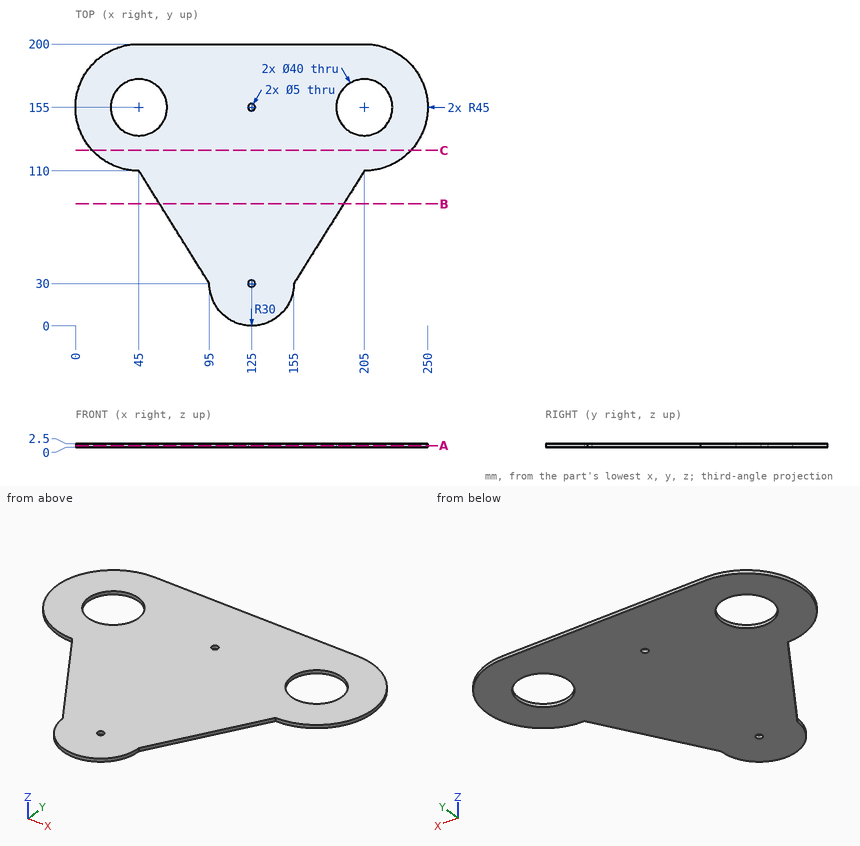
Source: three-view drawing plus pictorial views. Frame: mm from the lowest corner of the part. Round coordinates to 2 decimals unless told otherwise and drop trailing zeros. Write each loop counter-clockwise with the first axis right and the second up, starting at its lowest first coordinate (ties: lowest second). Pieces come first, ordered by that corner, then holes. Notation, with made-up numbers: M 63.5,27 L 72.5,27 A10 ccw 72.5,42 Z; hole C -22,-23 d3. An arc over 180 degrees is marked long. Use CSV: the item, a comma, the result in double quotes. Start each with the question number.
Q1. Cut plane C-C on y = 124.5. Output: boundary loops of the cut face in (x, z).
Q2. Line query: line 1 (Y direction, x = 125, z = 0.8); line 2 (Y direction, x = 206.5, z = 1.7) (3 decimals); line 3 (X direction, y = 169.5, z = 2.25). Output: solid intervals per line, ascending. Write a range as from..to.
Q3. Cut plane A-A on z = 1.25. Output: boundary loops of the cut face in (x, y), plus the area to 3 significant figures.
Q4. First-contact query: P1, Ø1.5, axis at x = 224.5, z = 0.5, coming from the -Y side; P2, Ø1.5, axis at x = 221, z = 2, coming from the +Y side. Flat tips, straight axial feed; report the tip coordinate or a pass-through.
Q5. Cut plane B-B on y = 86.5. Output: boundary loops of the cut face in (x, z), plus the area to 3 significant figures.
Results found:
1,outline,"M 11.91,0 L 238.09,0 L 238.09,2.5 L 11.91,2.5 Z"
2,line 1,"0..27.5, 32.5..152.5, 157.5..200"
2,line 2,"110.025..135.056, 174.944..199.975"
2,line 3,"2.4..31.23, 58.77..191.23, 218.77..247.6"
3,outline,"M 45,110 L 95,30 A30 ccw 155,30 L 205,110 A45 ccw 205,200 L 45,200 A45 ccw Z; hole C 45,155 d40; hole C 125,30 d5; hole C 125,155 d5; hole C 205,155 d40"
3,area,"28,400 mm^2"
4,P1,"y = 114.09"
4,P2,"y = 197.34"
5,outline,"M 59.69,0 L 190.31,0 L 190.31,2.5 L 59.69,2.5 Z"
5,area,"327 mm^2"
